```python
from build123d import *

# Parameters (mm, degrees)
CROQUIS1_R              = 45
SALIENTE_EXTRUIR1_DEPTH = 14.2
CROQUIS2_R              = 20
SALIENTE_EXTRUIR2_DEPTH = 44.2
CROQUIS3_R              = 25
SALIENTE_EXTRUIR3_DEPTH = 30
CROQUIS4_R              = 19
CORTAR_EXTRUIR1_DEPTH   = 24
CROQUIS5_R              = 15
CORTAR_EXTRUIR2_DEPTH   = 84
CHAFL_N1_SIZE           = 3.5
CHAFL_N1_SIZE2          = 3
CROQUIS6_R              = 6.25
CORTAR_EXTRUIR3_DEPTH   = 84


with BuildPart() as part:
    # Croquis1 → Saliente-Extruir1 (new body)
    with BuildSketch(Plane.XY):
        Circle(CROQUIS1_R)
    extrude(amount=SALIENTE_EXTRUIR1_DEPTH)

    # Croquis2 → Saliente-Extruir2 (add)
    with BuildSketch(Plane.XY.offset(14.2)):
        Circle(CROQUIS2_R)
    extrude(amount=SALIENTE_EXTRUIR2_DEPTH)

    # Croquis3 → Saliente-Extruir3 (add)
    with BuildSketch(Plane.XY.offset(58.4)):
        Circle(CROQUIS3_R)
    extrude(amount=SALIENTE_EXTRUIR3_DEPTH)

    # Croquis4 → Cortar-Extruir1 (cut)
    with BuildSketch(Plane.XY.offset(88.4)):
        Circle(CROQUIS4_R)
    extrude(amount=-CORTAR_EXTRUIR1_DEPTH, mode=Mode.SUBTRACT)

    # Croquis5 → Cortar-Extruir2 (cut)
    with BuildSketch(Plane.XY.offset(64.4)):
        Circle(CROQUIS5_R)
    extrude(amount=-CORTAR_EXTRUIR2_DEPTH, mode=Mode.SUBTRACT)

    # Chaflán1
    chafl_n1_edges = [part.edges().sort_by_distance(p)[0] for p in [
        (-15, 0, 0),
    ]]
    chafl_n1_side = [part.faces().sort_by_distance(p)[0] for p in [
        (-15, 0, 32.2),
    ]]
    chamfer(chafl_n1_edges, length=CHAFL_N1_SIZE, length2=CHAFL_N1_SIZE2, reference=chafl_n1_side[0])

    # Croquis6 → Cortar-Extruir3 (cut)
    with BuildSketch(Plane(origin=(0, 0, 0), x_dir=(-1, 0, 0), z_dir=(0, 0, -1))):
        with Locations((0, 32.5)):
            Circle(CROQUIS6_R)
        with Locations((32.5, 0)):
            Circle(CROQUIS6_R)
        with Locations((0, -32.5)):
            Circle(CROQUIS6_R)
        with Locations((-32.5, 0)):
            Circle(CROQUIS6_R)
    extrude(amount=-CORTAR_EXTRUIR3_DEPTH, mode=Mode.SUBTRACT)


solid = part.part
```
CAD build for the part. Positions are in the model's coordinates, mm. A direction names the side the tool comes from. Give positions to 0.01 mm unless a question says otherwise; leave off trailing zeros. Order: outer loops, then holes, each group sorted by start corner. A loop starts at its lowest first (then second) coordinate and runs counter-clockwise, first axis right, second up.
(1) Saw through at C-C, the plane y = -31. Give the cut face in (x, z).
(2) Flat gauge pins, fed straight in: pin 1 (25 mm diameter, centred on x = 2, y = -9, fed in from -Z); pin 2 (11 mm diameter, centred on x = 0, y = -32.5, fed in from +Z); pin 3 (1.5 mm diameter, centred on y = -5, z = 77, fed in from +X); pin 4 (10 mm diameter, centred on y = -12, z = 67.5, fed in from -X). Where does each tip first touch, or does it go through?
(3) Tool access for faces 4 (the cylindrical face through (-4.336, -19.524, 35.991)), 5 (the flat face through (14, 6, 64.4)), 6 (the cylindrical face through (-27.54, -3.8, 7)): list every direction of +Z, -Z, +X, -X, +Y, -Y with a clear straight run to the whole face (end or side of a thin tool).
(4) Saw through at A-A, the plane y = 0. State how many separate pieces and enclosed holes the cut face has, then the cut area to 3 significant figures.
(5) Drill centre lines: L1, parallel to Y at x = 0, z = 8; L2, parallel to Y at x = 0, z = 26; L3, parallel to Z at x = 21.5, y = -12. Where is each one in solid material? Low to high.
(6) Mould opens along Y. For faces 1 (the cylindrical face through (20.765, -39.923, 7.001)), 2 (the flat face through (-4, 19, 88.4)), 3 (the cylindrical face through (-5.96, -30.62, 7)) say: released by +Y, released by -Y, zero draft, split by the parting line, or undercut.
(7) Saw through at D-D, the plane z = 31.5. Give the cut face in (x, y).
Results found:
1. outline: (-32.62, 0) - (-6.07, 0) - (-6.07, 14.2) - (-32.62, 14.2) - close; (6.07, 0) - (32.62, 0) - (32.62, 14.2) - (6.07, 14.2) - close
2. pin 1: stops at z = 0
2. pin 2: passes through
2. pin 3: stops at x = 24.64
2. pin 4: stops at x = -24
3. face 4: none
3. face 5: +Z
3. face 6: +Z, -Z
4. separate pieces: 4
4. enclosed holes: 0
4. area: 1,340 mm2
5. L1: y = -45 to -38.75, -26.25 to -15, 15 to 26.25, 38.75 to 45
5. L2: y = -20 to -15, 15 to 20
5. L3: z = 0 to 14.2, 58.4 to 88.4
6. face 1: split by the parting line
6. face 2: zero draft
6. face 3: undercut
7. outline: circle Ø40 at (0, 0); hole circle Ø30 at (0, 0)
